For this review, take the finished solid that the model builds, in its own axes (mm). Face numbers are marked on the shaded views. A direction names the side the tool comes from. Give positions to 0.01 mm unless a question says otherwise; leave off trailing zeros. Loops run counter-clockwise (first coordinate to the right, second up) from the corner with the lowest first, then second, coordinate; pieces in that order, holes last. Notation, with made-up numbers: (-21.5, -13) - (4.5, -13) arc R32 ccw to (4.5, 17) - close; hole circle Ø6 at (-33.5, -12). An arc over 180 degrees is marked (long way). Answer as CSV lines item,"result".
from build123d import *

# Parameters (mm, degrees)
F0_R     = 21.7005672346
F0_R_2   = 10.1477344841
F1_DEPTH = 25
F2_COUNT = 12


with BuildPart() as f1:
    # F0 (on Front) → F1 (new body)
    with BuildSketch(Plane.XZ):
        with BuildLine():
            Line((0.0755267103, 61.0092692077), (-0.678219289, 61.0092692077))
            ThreePointArc((-0.678219289, 61.0092692077), (-1.4109604477, 60.9850584399), (-2.1430072202, 60.9450173375))
            ThreePointArc((-2.1430072202, 60.9450173375), (-2.9216954454, 60.8849691932), (-3.6987948092, 60.8070095215))
            ThreePointArc((-3.6987948092, 60.8070095215), (0.8564750407, -6.8151927129), (2.2940606408, 60.9450173375))
            Line((2.2940606408, 60.9450173375), (0.0755267103, 61.0092692077))
        make_face()
        with BuildLine():
            ThreePointArc((-1.4440762441, 52.1542261029), (17.2807567209, 45.3769750136), (25.1790579289, 27.0967304878))
            ThreePointArc((25.1790579289, 27.0967304878), (-17.1297033003, 8.816485962), (-1.4440762441, 52.1542261029))
        make_face(mode=Mode.SUBTRACT)
        with BuildLine():
            ThreePointArc((-1.4440762441, 52.1542261029), (-17.1297033003, 8.816485962), (25.1790579289, 27.0967304878))
            ThreePointArc((25.1790579289, 27.0967304878), (17.2807567209, 45.3769750136), (-1.4440762441, 52.1542261029))
        make_face()
        with Locations((0.0755267103, 27.0967304878)):
            Circle(F0_R, mode=Mode.SUBTRACT)
        with Locations((0.0755267103, 27.0967304878)):
            Circle(F0_R)
        with Locations((0.0755267103, 27.0967304878)):
            Circle(F0_R_2, mode=Mode.SUBTRACT)
        with BuildLine():
            ThreePointArc((-2.1430072202, 60.9450173375), (-1.4109604477, 60.9850584399), (-0.678219289, 61.0092692077))
            Line((-0.678219289, 61.0092692077), (0.0755267103, 61.0092692077))
            Line((0.0755267103, 61.0092692077), (2.2940606408, 60.9450173375))
            Line((2.2940606408, 60.9450173375), (2.3937216029, 64.932487905))
            Line((2.3937216029, 64.932487905), (0.7080621371, 66.9803842463))
            Line((0.7080621371, 66.9803842463), (-1.9470183179, 66.8063610792))
            Line((-1.9470183179, 66.8063610792), (-4.0409177, 66.0267961504))
            Line((-4.0409177, 66.0267961504), (-3.8679042053, 63.38712032))
            Line((-3.8679042053, 63.38712032), (-3.6987948092, 60.8070095215))
            ThreePointArc((-3.6987948092, 60.8070095215), (-2.9216954454, 60.8849691932), (-2.1430072202, 60.9450173375))
        make_face()
    extrude(amount=F1_DEPTH)

    # F2: F1 ×12 about axis
    f2_axis = Axis((0.0755267103, 0, 27.0967304878), (0, 1, 0))


with BuildPart() as f1_1:
    add(f1.part)
    for i in range(1, F2_COUNT):
        add(f1.part.rotate(f2_axis, i * 360 / F2_COUNT))


solid = f1_1.part
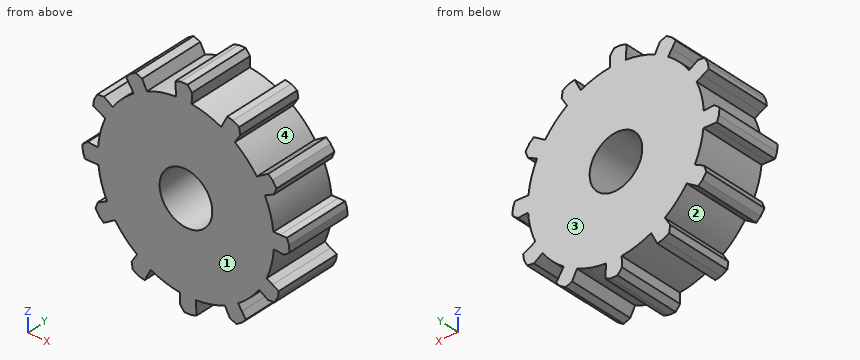
1) Insertion check: P1, Ø10, axis at x = -13, y = -9.5, coming from the -Z side; P2, Ø2, axis at y = -7, z = 35, coming from the +X side; P3, Ø1, axis at x = -28, z = 48, coming from the -Y side; P4, Ø1, axis at y = -14.5, z = 27.5, coming from the +X side. Each pin has a flat end and moves straight along its axis. Give the tip position at first contact, or say it passes through.
From the geometry:
P1,"stops at z = -8.68"
P2,"stops at x = 33.29"
P3,"passes through"
P4,"stops at x = 39.92"
2) Draft analysis for pull direction X (two halves, no side actions). For the marked faces 3 and 4, state which applies: pulls with the +X half, pulls with the -X half, needs draft (parallel to the pull), parting line crosses it, or undercut.
From the geometry:
face 3,"needs draft"
face 4,"undercut"
3) Consider section C-C on x = 25.5. Write out the cut boundary in (y, z), and give its area (3 significant figures).
From the geometry:
outline,"(-25, 4.64) - (0, 4.64) - (0, 49.55) - (-25, 49.55) - close"
area,"1,120 mm^2"
4) Consider section B-B on x = -6.5. Write out the cut boundary in (y, z).
From the geometry:
outline,"(-25, -6.18) - (0, -6.18) - (0, 19.37) - (-25, 19.37) - close; (-25, 34.83) - (0, 34.83) - (0, 60.37) - (-25, 60.37) - close"
5) Wall thickness on line 1 (Z direction, x = 6, y = -19.5); line 2 (X direction, y = -19, z = 46.5); line 3 (X direction, y = -21.5, z = 25): over which ranges is each line inside the solid? List them lowest first. Write a range as from..to.
From the geometry:
line 1,"z = -6.3..18.86, 35.34..60.5"
line 2,"x = -34.68..-29.04, -27.75..34.93"
line 3,"x = -39.61..-9.85, 10..38.18"
6) Consider section D-D on z = 53. Write out the cut boundary in (x, y).
From the geometry:
outline,"(-21.83, -25) - (21.98, -25) - (21.98, 0) - (-21.83, 0) - close"
7) Machinability: for the marked faces 1 and 2, which of the approach directions +Z, -Z, +X, -X, +Y, -Y give a long, thin tool a straight path to every point of the face, cutting with its end or side? Answer none if there is none.
From the geometry:
face 1,"+Z, -Z, +X, -X, -Y"
face 2,"+Y, -Y"
8) Consider section A-A on z = 21.5. Write out the cut boundary in (x, y).
From the geometry:
outline,"(-33.38, -25) - (-8.39, -25) - (-8.39, 0) - (-33.38, 0) - close; (8.54, -25) - (33.53, -25) - (33.53, 0) - (8.54, 0) - close"
